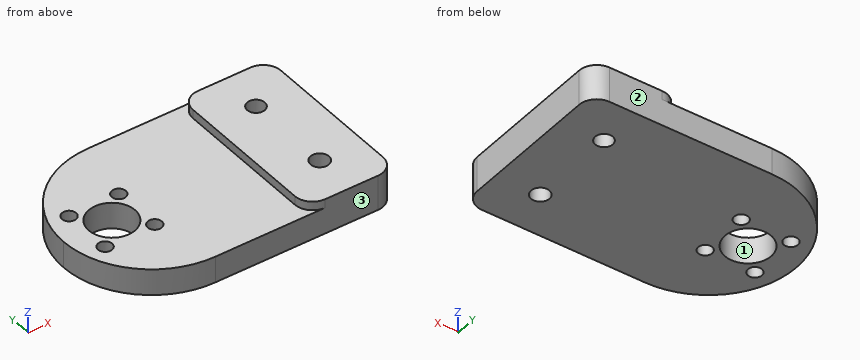
from build123d import *

# Parameters (mm, degrees)
F0_W     = 61
F0_H     = 40
F0_R     = 1.6
F0_R_2   = 2.1
F0_R_3   = 5.25
F0_R_4   = 2
F1_DEPTH = 6
F2_DEPTH = 77
F3_R     = 19.99999
F4_W     = 20
F4_H     = 40
F4_R     = 2.1
F4_R_2   = 2
F5_DEPTH = 2
F6_R     = 4


# Not quite as in the source:
# - a fillet or chamfer is up to 0.001 mm smaller than in the source, because OpenCascade refuses the exact size
# - an extrude ends at something that could not be found from the text; its depth is read off the source's solid


with BuildPart() as f1:
    # F0 (on Top) → F1 (new body)
    with BuildSketch(Plane.XY):
        Rectangle(F0_W, F0_H)
        with Locations((-25.15, -5.65)):
            Circle(F0_R, mode=Mode.SUBTRACT)
        with Locations((-13.85, -5.65)):
            Circle(F0_R, mode=Mode.SUBTRACT)
        with Locations((20.5, -10)):
            Circle(F0_R_2, mode=Mode.SUBTRACT)
        with Locations((-19.5, 0)):
            Circle(F0_R_3, mode=Mode.SUBTRACT)
        with Locations((-25.15, 5.65)):
            Circle(F0_R, mode=Mode.SUBTRACT)
        with Locations((-13.85, 5.65)):
            Circle(F0_R, mode=Mode.SUBTRACT)
        with Locations((20.5, 10)):
            Circle(F0_R_4, mode=Mode.SUBTRACT)
    extrude(amount=F1_DEPTH)

    # F0 (on Top) → F2 (cut, through all)
    with BuildSketch(Plane.XY):
        Rectangle(F0_W, F0_H)
        with Locations((-25.15, -5.65)):
            Circle(F0_R, mode=Mode.SUBTRACT)
        with Locations((-13.85, -5.65)):
            Circle(F0_R, mode=Mode.SUBTRACT)
        with Locations((20.5, -10)):
            Circle(F0_R_2, mode=Mode.SUBTRACT)
        with Locations((-19.5, 0)):
            Circle(F0_R_3, mode=Mode.SUBTRACT)
        with Locations((-25.15, 5.65)):
            Circle(F0_R, mode=Mode.SUBTRACT)
        with Locations((-13.85, 5.65)):
            Circle(F0_R, mode=Mode.SUBTRACT)
        with Locations((20.5, 10)):
            Circle(F0_R_4, mode=Mode.SUBTRACT)
    extrude(amount=-F2_DEPTH, mode=Mode.SUBTRACT)

    # F3 (radius 20 in the source; OpenCascade refuses exactly that, so slightly less here)
    f3_edges = [f1.edges().sort_by_distance(p)[0] for p in [
        (-30.5, -20, 3),
        (-30.5, 20, 3),
    ]]
    fillet(f3_edges, radius=F3_R)

    # F4 (on face) → F5 (join)
    with BuildSketch(Plane.XY.offset(6)):
        with Locations((20.5, 0)):
            Rectangle(F4_W, F4_H)
        with Locations((20.5, -10)):
            Circle(F4_R, mode=Mode.SUBTRACT)
        with Locations((20.5, 10)):
            Circle(F4_R_2, mode=Mode.SUBTRACT)
    extrude(amount=F5_DEPTH)

    # F6
    f6_edges = [f1.edges().sort_by_distance(p)[0] for p in [
        (10.5, -20, 7),
        (30.5, -20, 4),
        (10.5, 20, 7),
        (30.5, 20, 4),
    ]]
    fillet(f6_edges, radius=F6_R)


solid = f1.part
The listing builds one solid part. Answer for the finished solid, in the listing's coordinates (mm). Face numbers are marked on the shaded views. Coordinates: 2 decimals unless noted, no trailing zeros. Loops run counter-clockwise (first coordinate to the right, second up) from the corner with the lowest first, then second, coordinate; pieces in that order, holes last. Notation, with made-up numbers: (41, 80.25) -> (86, 80.25) arc R20 cw to (86, 118.25) -> close; hole circle Ø2 at (87, -0.5). An arc over 180 degrees is marked (long way). Answer in a Markdown table with one row per item. Add a question column.
1. The part is cut by section A-A, the plane x = 20.5. Write down the section's boundary in (y, z).
2. The part is cut by section D-D, the plane z = 4. Count the separate pieces of the cut face and the enclosed holes in it, then the cut area to 3 significant figures.
3. Consider line 1 (Y direction, x = -13.85, z = 1.65); line 2 (Y direction, x = -25.15, z = 3.3); line 3 (Z direction, x = -11.5, y = 8). Determine where each line is inside the solid, lowest interval first. Write a range as [from, to].
4. Determine the mould class of the marked faces 1, 2 and 3 for opening direction Y: +Y half, -Y half, draft (parallel to the pull), parting line (faces both ways), or undercut.
5. The part is cut by section C-C, the plane x = -17.5. Write down the section's boundary in (y, z) (3 decimals).
6. The part is cut by section B-B, the plane y = -10. Write down the section's boundary in (x, z).
7. Flat-ended cylindrical pins translate along their axes: P1, Ø20, axis at x = -18, y = -5.5, coming from the +Z side; P2, Ø0.6, axis at y = -3, z = 7.5, coming from the -X side; P3, Ø4, axis at y = 8.5, z = 1.5, coming from the -X side. Find the tip coordinate at first contact, or state that the pin passes through.
Answer below:
| question | item | result |
|---|---|---|
| 1 | outline | (-20, 0) -> (-12.1, 0) -> (-12.1, 8) -> (-20, 8) -> close; (-7.9, 0) -> (8, 0) -> (8, 8) -> (-7.9, 8) -> close; (12, 0) -> (20, 0) -> (20, 8) -> (12, 8) -> close |
| 2 | separate pieces | 1 |
| 2 | enclosed holes | 7 |
| 2 | area | 2,120 mm2 |
| 3 | line 1 | [-19.72, -7.25], [-4.05, 4.05], [7.25, 19.72] |
| 3 | line 2 | [-13.62, -7.25], [-4.05, 4.05], [7.25, 13.62] |
| 3 | line 3 | [0, 6] |
| 4 | face 1 | undercut |
| 4 | face 2 | +Y half |
| 4 | face 3 | -Y half |
| 5 | outline | (-18.735, 0) -> (-4.854, 0) -> (-4.854, 6) -> (-18.735, 6) -> close; (4.854, 0) -> (18.735, 0) -> (18.735, 6) -> (4.854, 6) -> close |
| 6 | outline | (-27.82, 0) -> (18.4, 0) -> (18.4, 8) -> (10.5, 8) -> (10.5, 6) -> (-27.82, 6) -> close; (22.6, 0) -> (30.5, 0) -> (30.5, 8) -> (22.6, 8) -> close |
| 7 | P1 | z = 6 |
| 7 | P2 | x = 10.5 |
| 7 | P3 | x = -29.41 |
